Check sheet for the modelled part. Datum: model origin and axes. Units: mm. Face numbers are marked on the shaded views. A direction names the side the tool comes from. Give positions to 0.01 mm unless a question says otherwise; leave off trailing zeros. Write each loop counter-clockwise with the first axis right and the second up, starting at its lowest first coordinate (ties: lowest second). Pieces come first, ordered by that corner, then holes. Notation, with made-up numbers: (25, 33) -> (56, 33) arc R27 ccw to (56, 51) -> close; hole circle Ø2 at (41, 46). An arc over 180 degrees is marked (long way). Answer as a JSON object with one key per item and string values.
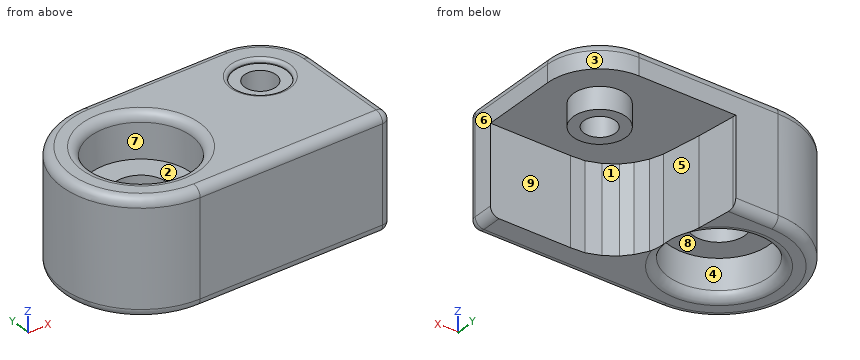
from build123d import *

# Parameters (mm, degrees)
CYLINDER020_R     = 1.8
CYLINDER020_DEPTH = 7
CYLINDER021_R     = 3
CYLINDER021_DEPTH = 7
PAD_DEPTH         = 30
BOX002_W          = 10
BOX002_H          = 10
BOX002_DEPTH      = 10
BOX003_W          = 17
BOX003_H          = 10
BOX003_DEPTH      = 10
CYLINDER018_R     = 5.75
CYLINDER018_DEPTH = 10
CYLINDER017_R     = 3
CYLINDER017_DEPTH = 10
CYLINDER016_R     = 5.75
CYLINDER016_DEPTH = 10
CYLINDER015_R     = 3
CYLINDER015_DEPTH = 10
BOX_W             = 22
BOX_H             = 18
BOX_DEPTH         = 13
CYLINDER_R        = 9
CYLINDER_DEPTH    = 13
FILLET_R          = 6
FILLET001_R       = 1
FILLET002_R       = 1
FILLET003_R       = 1
CYLINDER019_R     = 3
CYLINDER019_DEPTH = 3
FILLET004_R       = 0.4


with BuildPart() as m3cut:
    # Cylinder020 → Cylinder020 (new body)
    with BuildSketch(Plane(origin=(-4.5, -22, 62.5), x_dir=(1, 0, 0), z_dir=(0, 0, 1))):
        Circle(CYLINDER020_R)
    extrude(amount=CYLINDER020_DEPTH)


with BuildPart() as fusion009:
    # Cylinder021 → Cylinder021 (new body)
    with BuildSketch(Plane(origin=(-4.5, -22, 67.5), x_dir=(1, 0, 0), z_dir=(0, 0, 1))):
        Circle(CYLINDER021_R)
    extrude(amount=CYLINDER021_DEPTH)

    # Fusion009: union m3Cut
    add(m3cut.part)


with BuildPart() as body:
    # Sketch → Pad (new body)
    with BuildSketch(Plane.XY):
        Polygon((-15.594093, -16.374565), (-15.071085, -20.857502), (-14.364655, -25.305099), (-13.862565, -26.78348), (-13.081532, -28.094496), (-12.161032, -29.126572), (-10.822123, -30.019178), (-9.315848, -30.577057), (-7.725893, -30.688633), (7.476312, -30.688633), (-15.876865, 6.281797), (-15.876865, -11.843776), align=None)
    extrude(amount=PAD_DEPTH)

    # Box002 → Box002 (join)
    with BuildSketch(Plane.XY):
        with Locations((5, 5)):
            Rectangle(BOX002_W, BOX002_H)
    extrude(amount=BOX002_DEPTH)


with BuildPart() as body_1:
    # Body placement: moved
    add(body.part.moved(Location((0, 0, 35))))


with BuildPart() as firstcuts:
    # Box003 → Box003 (new body)
    with BuildSketch(Plane(origin=(-10, -24, 55), x_dir=(1, 0, 0), z_dir=(0, 0, 1))):
        with Locations((8.5, 5)):
            Rectangle(BOX003_W, BOX003_H)
    extrude(amount=BOX003_DEPTH)

    # Fusion007: union Body
    add(body_1.part)


with BuildPart() as obj1:
    # Cylinder018 → Cylinder018 (new body)
    with BuildSketch(Plane(origin=(-23, 0, 69), x_dir=(1, 0, 0), z_dir=(0, 0, 1))):
        Circle(CYLINDER018_R)
    extrude(amount=CYLINDER018_DEPTH)


with BuildPart() as fusion005:
    # Cylinder017 → Cylinder017 (new body)
    with BuildSketch(Plane(origin=(-23, 0, 65), x_dir=(1, 0, 0), z_dir=(0, 0, 1))):
        Circle(CYLINDER017_R)
    extrude(amount=CYLINDER017_DEPTH)

    # Fusion005: union obj1
    add(obj1.part)


with BuildPart() as fusion005_1:
    # Fusion005 placement: moved
    add(fusion005.part.moved(Location((2.5, -25, -19.5))))


with BuildPart() as obj2:
    # Cylinder016 → Cylinder016 (new body)
    with BuildSketch(Plane(origin=(-23, 0, 69), x_dir=(1, 0, 0), z_dir=(0, 0, 1))):
        Circle(CYLINDER016_R)
    extrude(amount=CYLINDER016_DEPTH)


with BuildPart() as antennacuts:
    # Cylinder015 → Cylinder015 (new body)
    with BuildSketch(Plane(origin=(-23, 0, 65), x_dir=(1, 0, 0), z_dir=(0, 0, 1))):
        Circle(CYLINDER015_R)
    extrude(amount=CYLINDER015_DEPTH)

    # Fusion004: union obj2
    add(obj2.part)


with BuildPart() as antennacuts_1:
    # Fusion004 placement: moved
    add(antennacuts.part.moved(Location((2.5, -25, -6))))

    # Fusion006: union Fusion005
    add(fusion005_1.part)


with BuildPart() as cube:
    # Box → Box (new body)
    with BuildSketch(Plane(origin=(-20.5, -34, 56), x_dir=(1, 0, 0), z_dir=(0, 0, 1))):
        with Locations((11, 9)):
            Rectangle(BOX_W, BOX_H)
    extrude(amount=BOX_DEPTH)


with BuildPart() as cut001:
    # Cylinder → Cylinder (new body)
    with BuildSketch(Plane(origin=(-20.5, -25, 56), x_dir=(1, 0, 0), z_dir=(0, 0, 1))):
        Circle(CYLINDER_R)
    extrude(amount=CYLINDER_DEPTH)

    # Fusion: union Cube
    add(cube.part)


with BuildPart() as cut001_1:
    # Fusion placement: moved
    add(cut001.part.moved(Location((0, 0, -1))))

    # Fillet
    fillet_edges = [cut001_1.edges().sort_by_distance(p)[0] for p in [
        (1.5, -16, 61.5),
    ]]
    fillet(fillet_edges, radius=FILLET_R)

    # Fillet001
    fillet001_edges = [cut001_1.edges().sort_by_distance(p)[0] for p in [
        (-12.5, -16, 55),
        (-9.5, -34, 55),
        (1.5, -28, 55),
        (-12.5, -16, 68),
        (1.5, -28, 68),
        (1.5, -34, 61.5),
        (-9.5, -34, 68),
        (-29.5, -25, 55),
        (-29.5, -25, 68),
    ]]
    fillet(fillet001_edges, radius=FILLET001_R)

    # Cut: cut antennaCuts
    add(antennacuts_1.part, mode=Mode.SUBTRACT)

    # Fillet002
    fillet002_edges = [cut001_1.edges().sort_by_distance(p)[0] for p in [
        (-16.434136, -29.065864, 68),
        (-16.434136, -20.934136, 68),
    ]]
    fillet(fillet002_edges, radius=FILLET002_R)

    # Fillet003
    fillet003_edges = [cut001_1.edges().sort_by_distance(p)[0] for p in [
        (-16.434136, -29.065864, 55),
        (-16.434136, -20.934136, 55),
        (-26.25, -25, 55),
    ]]
    fillet(fillet003_edges, radius=FILLET003_R)

    # Cut001: cut firstCuts
    add(firstcuts.part, mode=Mode.SUBTRACT)


with BuildPart() as fillet004:
    # Cylinder019 → Cylinder019 (new body)
    with BuildSketch(Plane(origin=(-4.5, -22, 62.5), x_dir=(1, 0, 0), z_dir=(0, 0, 1))):
        Circle(CYLINDER019_R)
    extrude(amount=CYLINDER019_DEPTH)

    # Fusion008: union Cut001
    add(cut001_1.part)

    # Cut002: cut Fusion009
    add(fusion009.part, mode=Mode.SUBTRACT)

    # Fillet004
    fillet004_edges = [fillet004.edges().sort_by_distance(p)[0] for p in [
        (-7.5, -22, 68),
    ]]
    fillet(fillet004_edges, radius=FILLET004_R)


solid = fillet004.part
1. Access from +Z, -Z, +X, -X, +Y, -Y to the whole of each face (thin tool, end or side, straight path). Record for the marked faces 1, 2, 3, 4 and 5.
Determined:
{"face 1": "-Z, +X, +Y", "face 2": "+Z", "face 3": "+Z, -Z, +X, +Y", "face 4": "-Z", "face 5": "-Z, +Y"}
2. Sectioned sample at D-D, the plane y = -23. State how many separate pieces and enclosed holes the cut face has, plus the area to 3 significant figures.
Determined:
{"separate pieces": "3", "enclosed holes": "0", "area": "114 mm^2"}
3. Sectioned sample at C-C, the plane z = 58.25. Enter the section's corners in (x, y), plus the area to 3 significant figures.
Determined:
{"outline": "(-20.5, -34) -> (0.5, -34) arc R1 ccw to (1.5, -33) -> (1.5, -30.69) -> (-7.73, -30.69) -> (-9.32, -30.58) -> (-10.82, -30.02) -> (-12.16, -29.13) -> (-13.08, -28.09) -> (-13.86, -26.78) -> (-14.36, -25.31) -> (-15.07, -20.86) -> (-15.59, -16.37) -> (-15.62, -16) -> (-20.5, -16) arc R9 ccw to start; hole circle Ø11.5 at (-20.5, -25)", "area": "189 mm^2"}
4. Go/stop test with flat-tipped pins: P1, Ø3, axis at y = -28.5, z = 64.5, coming from the -X side; P2, Ø7, axis at x = -4.5, y = -22, coming from the -Z side; P3, Ø3, axis at x = -5, z = 59.5, coming from the +Y side; P4, Ø6.5, axis at x = -5, y = -21, coming from the +Z side. Record where each tip stops, or that it passes through.
Determined:
{"P1": "x = -29.27", "P2": "z = 62.5", "P3": "y = -30.69", "P4": "z = 68"}
5. Sectioned sample at B-B, the plane z = 66.5. Enter the section's corners in (x, y), plus the area to 3 significant figures.
Determined:
{"outline": "(-20.5, -34) -> (0.5, -34) arc R1 ccw to (1.5, -33) -> (1.5, -22) arc R6 ccw to (-4.5, -16) -> (-20.5, -16) arc R9 ccw to start; hole circle Ø11.5 at (-20.5, -25); hole circle Ø3.6 at (-4.5, -22)", "area": "401 mm^2"}
6. Mould release check, pull along X, two halves, no side actions. Record for the marked faces 6, 7, 8 and 9: released by +X, released by -X, zero draft, split by the parting line, or undercut.
Determined:
{"face 6": "released by +X", "face 7": "undercut", "face 8": "undercut", "face 9": "zero draft"}
7. Sectioned sample at A-A, the plane z = 63.5. Enter the section's corners in (x, y).
Determined:
{"outline": "(-20.5, -34) -> (0.5, -34) arc R1 ccw to (1.5, -33) -> (1.5, -30.69) -> (-7.73, -30.69) -> (-9.32, -30.58) -> (-10.82, -30.02) -> (-12.16, -29.13) -> (-13.08, -28.09) -> (-13.86, -26.78) -> (-14.36, -25.31) -> (-15.07, -20.86) -> (-15.59, -16.37) -> (-15.62, -16) -> (-20.5, -16) arc R9 ccw to start; circle Ø6 at (-4.5, -22); hole circle Ø11.5 at (-20.5, -25); hole circle Ø3.6 at (-4.5, -22)"}
8. Scan lines: L1, parallel to X at y = -22, z = 67.6; L2, parallel to Y at x = -4.5, z = 63; L3, parallel to Y at x = -20.5, z = 65.75. Record each from-to range of solid material in increasing order. Write a range as [from, to].
Determined:
{"L1": "[-28.77, -25.64], [-15.36, -7.5], [-1.5, 1.3]", "L2": "[-34, -30.69], [-25, -23.8], [-20.2, -19]", "L3": "[-34, -30.75], [-19.25, -16]"}
